Geometry: final body of the model. Coordinates: model frame, mm. A direction names the side the tool comes from. Give positions to 0.01 mm unless a question says otherwise; leave off trailing zeros. Loops run counter-clockwise (first coordinate to the right, second up) from the corner with the lowest first, then second, coordinate; pieces in that order, holes last.
from build123d import *

# Parameters (mm, degrees)
BOSS_EXTRUDE1_DEPTH     = 4
SKETCH3_W               = 20
SKETCH3_H               = 25
CUT_EXTRUDE1_DEPTH      = 2
CUT_EXTRUDE2_DEPTH      = 78.081938119
CUT_EXTRUDE2_DEPTH_BACK = 78.081938119
CUT_EXTRUDE3_DEPTH      = 78.081938119
LPATTERN1_COUNT         = 26
LPATTERN1_PITCH         = 1.0025
CUT_EXTRUDE4_DEPTH      = 78.081938119
CUT_EXTRUDE5_DEPTH      = 78.081938119
FILLET1_R               = 10
FILLET2_R               = 2
FILLET3_R               = 1
FILLET4_R               = 0.5
SKETCH9_R               = 1.5
CUT_EXTRUDE6_DEPTH      = 77.824835617


with BuildPart() as part:
    # Sketch1 → Boss-Extrude1 (new, symmetric)
    with BuildSketch(Plane.XY):
        Polygon((0, 0), (-20, 30.005392849), (-20, 60.135392849), (-21.435566599, 73.055886204), (-16.466146078, 73.608027203), (-14.000284373, 51.414595156), (-14.000284373, 50.014595156), (0, 40.028289364), align=None)
    extrude(amount=BOSS_EXTRUDE1_DEPTH, both=True)

    # Sketch3 → Cut-Extrude1 (cut, symmetric)
    with BuildSketch(Plane.XY):
        with Locations((-24.000284373, 62.514595156)):
            Rectangle(SKETCH3_W, SKETCH3_H)
    extrude(amount=CUT_EXTRUDE1_DEPTH, both=True, mode=Mode.SUBTRACT)

    # Sketch5 → Cut-Extrude2 (cut, two sides: drawn at the far end of the back side and taken through both)
    with BuildSketch(Plane.XY.offset(4).offset(-CUT_EXTRUDE2_DEPTH_BACK)):
        with BuildLine():
            Line((91.496624596, 102.650757811), (0, 34.028289364))
            ThreePointArc((0, 34.028289364), (-2, 30.028289364), (0, 26.028289364))
            Line((0, 26.028289364), (91.496624596, -42.594179083))
            Line((91.496624596, -42.594179083), (320.238186086, -42.594179083))
            Line((320.238186086, -42.594179083), (320.238186086, 102.650757811))
            Line((320.238186086, 102.650757811), (91.496624596, 102.650757811))
        make_face()
    extrude(amount=CUT_EXTRUDE2_DEPTH + CUT_EXTRUDE2_DEPTH_BACK, mode=Mode.SUBTRACT)

    # Sketch6 → Cut-Extrude3 (cut, through all)
    with BuildSketch(Plane.XY.offset(4)):
        Polygon((0, 26.028289364), (-0.5, 25.028289364), (0, 25.028289364), align=None)
    cut_extrude3 = extrude(amount=-CUT_EXTRUDE3_DEPTH, mode=Mode.SUBTRACT)

    # LPattern1: Cut-Extrude3 ×26
    with Locations(*[(0, -i * LPATTERN1_PITCH, 0) for i in range(1, LPATTERN1_COUNT)]):
        add(cut_extrude3, mode=Mode.SUBTRACT)

    # Sketch7 → Cut-Extrude4 (cut, through all)
    with BuildSketch(Plane.XY.offset(4)):
        with BuildLine():
            Line((-20, 45.005392849), (-20, 30.005392849))
            Line((-20, 30.005392849), (-6.955074875, 10.434487696))
            ThreePointArc((-6.955074875, 10.434487696), (-12.476218242, 28.097776313), (-20, 45.005392849))
        make_face()
    extrude(amount=-CUT_EXTRUDE4_DEPTH, mode=Mode.SUBTRACT)

    # Sketch8 → Cut-Extrude5 (cut, through all)
    with BuildSketch(Plane.XY.offset(4)):
        with BuildLine():
            Line((-14.004117633, 45.104021749), (-5, 38.681447059))
            Line((-5, 38.681447059), (-5, 17.744021749))
            ThreePointArc((-5, 17.744021749), (-9.031897039, 29.772645882), (-14.004117633, 41.444021749))
            Line((-14.004117633, 41.444021749), (-14.004117633, 45.104021749))
        make_face()
    extrude(amount=-CUT_EXTRUDE5_DEPTH, mode=Mode.SUBTRACT)

    # Fillet1
    fillet1_edges = [part.edges().sort_by_distance(p)[0] for p in [
        (0, 40.028289364, 0),
        (-20, 45.005392849, 0),
        (-6.955074875, 10.434487696, 0),
    ]]
    fillet(fillet1_edges, radius=FILLET1_R)

    # Fillet2
    fillet2_edges = [part.edges().sort_by_distance(p)[0] for p in [
        (-21.435566599, 73.055886204, 3),
        (-16.466146078, 73.608027203, 3),
        (-14.000284373, 50.014595156, 3),
        (-21.435566599, 73.055886204, -3),
        (-16.466146078, 73.608027203, -3),
        (-14.000284373, 50.014595156, -3),
    ]]
    fillet(fillet2_edges, radius=FILLET2_R)

    # Fillet3
    fillet3_edges = [part.edges().sort_by_distance(p)[0] for p in [
        (-14.004117633, 41.444021749, 0),
        (-14.004117633, 45.104021749, 0),
        (-5, 38.681447059, 0),
    ]]
    fillet(fillet3_edges, radius=FILLET3_R)

    # Fillet4
    fillet4_edges = [part.edges().sort_by_distance(p)[0] for p in [
        (-5, 17.744021749, 0),
    ]]
    fillet(fillet4_edges, radius=FILLET4_R)

    # Sketch9 → Cut-Extrude6 (cut, through all)
    with BuildSketch(Plane.XY.offset(4)):
        with Locations((-18.416383851, 68.521557639)):
            Circle(SKETCH9_R)
        with Locations((-16.915664614, 55.014672662)):
            Circle(SKETCH9_R)
    extrude(amount=-CUT_EXTRUDE6_DEPTH, mode=Mode.SUBTRACT)


solid = part.part
Item 1: Draft query along Z for faces 1 (the face through (-18, 62, -2)), 2 (the face through (-20, 52, 3)). Return one class per face: +Z half, -Z half, draft (parallel to the pull), parting line (faces both ways), or undercut.
Values follow:
face 1: undercut
face 2: draft
Item 2: Section query B-B on x = -8. Return loops of the section in (y, z), plus the area to 3 significant figures.
Values follow:
outline: (14.4, -4) - (26.98, -4) - (26.98, 4) - (14.4, 4) - close; (40.82, -4) - (45.73, -4) - (45.73, 4) - (40.82, 4) - close
area: 140 mm2
Item 3: Section query C-C on z = 3. Give the number of separate pieces and of enclosed holes in the cut face, plus the area to 3 significant figures.
Values follow:
separate pieces: 1
enclosed holes: 3
area: 491 mm2
Item 4: Pin query (flat end, axial travel): pin 1 (1.5 mm diameter, centred on x = -5, z = -1.5, fed in from +Y). Return the tip coordinate at first contact, or that it passes through.
Values follow:
pin 1: stops at y = 44.13
Item 5: Section query A-A on y = 40. Return loops of the section in (x, z).
Values follow:
outline: (-17.53, -4) - (-13.33, -4) - (-13.33, 4) - (-17.53, 4) - close; (-6.85, -4) - (-1.41, -4) - (-1.41, 4) - (-6.85, 4) - close
Item 6: Set-up query: faces 3 (the face through (-13.448, 44.058, -0.056)), 4 (the face through (-13.772, 50.117, -2.986)). Return all of +Z, -Z, +X, -X, +Y, -Y with unobstructed straight access to the full face (end or side cutting, diameter ignored); none if empty.
Values follow:
face 3: +Z, -Z
face 4: +Z, -Z, +X, +Y
Item 7: Ray query, probe 1 along Z at (x, y) = (-17.25, 60.5); probe 2 along X at (y, z) = (54.5, 3.5); probe 3 along X at (y, z) = (23.5, 3.5). Return the intervals inside material, ascending.
Values follow:
probe 1: z = -4 to -2, 2 to 4
probe 2: x = -20 to -18.32, -15.51 to -14.34
probe 3: x = -10.82 to -6.8, -5 to -0.26
